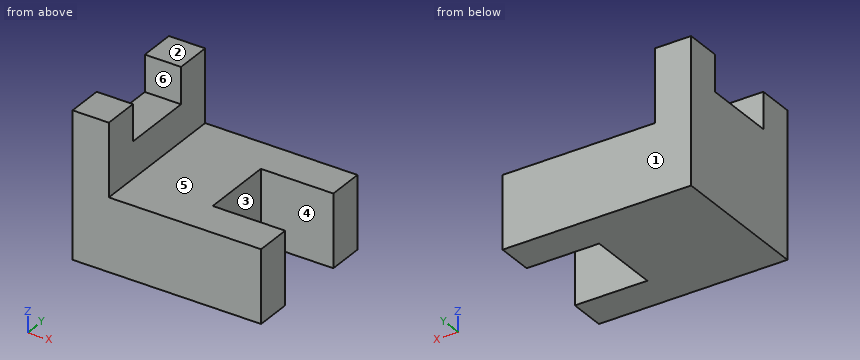
```python
from build123d import *

# Parameters (mm, degrees)
F1_DEPTH = 25.4
F2_W     = 12.7
F2_H     = 12.7
F3_DEPTH = 12.701
F4_W     = 6.35
F4_H     = 12.7
F5_DEPTH = 6.35


with BuildPart() as f1:
    # F0 (on Front) → F1 (new body)
    with BuildSketch(Plane.XZ):
        Polygon((0, 25.4), (0, 0), (33.02, 0), (33.02, 12.7), (6.35, 12.7), (6.35, 25.4), align=None)
    extrude(amount=F1_DEPTH)

    # F2 (on face) → F3 (cut, through all)
    with BuildSketch(Plane.XY.offset(12.7)):
        with Locations((26.67, -12.7)):
            Rectangle(F2_W, F2_H)
    extrude(amount=-F3_DEPTH, mode=Mode.SUBTRACT)

    # F4 (on face) → F5 (cut)
    with BuildSketch(Plane.XY.offset(25.4)):
        with Locations((3.175, -12.7)):
            Rectangle(F4_W, F4_H)
    extrude(amount=-F5_DEPTH, mode=Mode.SUBTRACT)


solid = f1.part
```
Read the model definition and answer for the solid it produces. Units are mm, in the model's axes. Face numbers are marked on the shaded views. A direction names the side the tool comes from. Give positions to 0.01 mm unless a question says otherwise; leave off trailing zeros. Loops run counter-clockwise (first coordinate to the right, second up) from the corner with the lowest first, then second, coordinate; pieces in that order, holes last.
Item 1: The part is cut by section D-D (x = 4). Write down the section's boundary in (y, z), and give its area (3 significant figures).
Item 2: The part is cut by section B-B (z = 3.5). Write down the section's boundary in (x, y), and give its area (3 significant figures).
Item 3: The part is cut by section A-A (x = 23). Write down the section's boundary in (y, z).
Item 4: Each of these flat-tipped pins is pushed along its axis until it touches: pin 1 Ø1 at (x, y) = (20.5, -17) entering from +Z; pin 2 Ø1.5 at (y, z) = (-15.5, 3) entering from +X; pin 3 Ø10 at (y, z) = (-8, 19.5) entering from +X. Where does it stop, or does it pass through?
Item 5: For the marked faces 4, 5 and 6, determine the directions among +Z, -Z, +X, -X, +Y, -Y from which every point of the face is accessible in a straight line to the end or side of a thin tool.
Item 6: The part is cut by section C-C (y = -16.25). Write down the section's boundary in (x, z), and give its area (3 significant figures).
Item 7: Find the intervals of material crossed by line 1 along Y through (x, z) = (26.5, 11.5); line 2 along Z through (x, y) = (29, -20.5); line 3 along X through (y, z) = (-23, 19.25), in increasing order.
Item 8: The mould has two halves that part along Y. Classify the marked faces 1, 2 and 3: released by +Y, released by -Y, zero draft, split by the parting line, or undercut.
Taken from the geometry:
1. outline: (-25.4, 0) - (0, 0) - (0, 25.4) - (-6.35, 25.4) - (-6.35, 19.05) - (-19.05, 19.05) - (-19.05, 25.4) - (-25.4, 25.4) - close
1. area: 565 mm2
2. outline: (0, -25.4) - (33.02, -25.4) - (33.02, -19.05) - (20.32, -19.05) - (20.32, -6.35) - (33.02, -6.35) - (33.02, 0) - (0, 0) - close
2. area: 677 mm2
3. outline: (-25.4, 0) - (-19.05, 0) - (-19.05, 12.7) - (-25.4, 12.7) - close; (-6.35, 0) - (0, 0) - (0, 12.7) - (-6.35, 12.7) - close
4. pin 1: stops at z = 12.7
4. pin 2: stops at x = 20.32
4. pin 3: stops at x = 6.35
5. face 4: +Z, -Z, +X
5. face 5: +Z, +X, +Y, -Y
5. face 6: +Z, +X, -X
6. outline: (0, 0) - (20.32, 0) - (20.32, 12.7) - (6.35, 12.7) - (6.35, 19.05) - (0, 19.05) - close
6. area: 298 mm2
7. line 1: y = -25.4 to -19.05, -6.35 to 0
7. line 2: z = 0 to 12.7
7. line 3: x = 0 to 6.35
8. face 1: released by +Y
8. face 2: zero draft
8. face 3: undercut
